Can you work these out from the drawing? Everything is in mm from the part's minimum corner. A direction names the side the tool comes from. Round coordinates to 2 decimals unless told otherwise and drop trailing zeros. Write each loop counter-clockwise with the first axis right and the second up, starting at its lowest first coordinate (ties: lowest second). Pieces come first, ordered by that corner, then holes. Notation, with made-up numbers: M -24.75,-5.75 L 26.25,-5.75 A20 ccw 26.25,7.25 Z; hole C 42.25,54 d11. An arc over 180 degrees is marked long. Use a Markdown table: item, result. Add a question column.
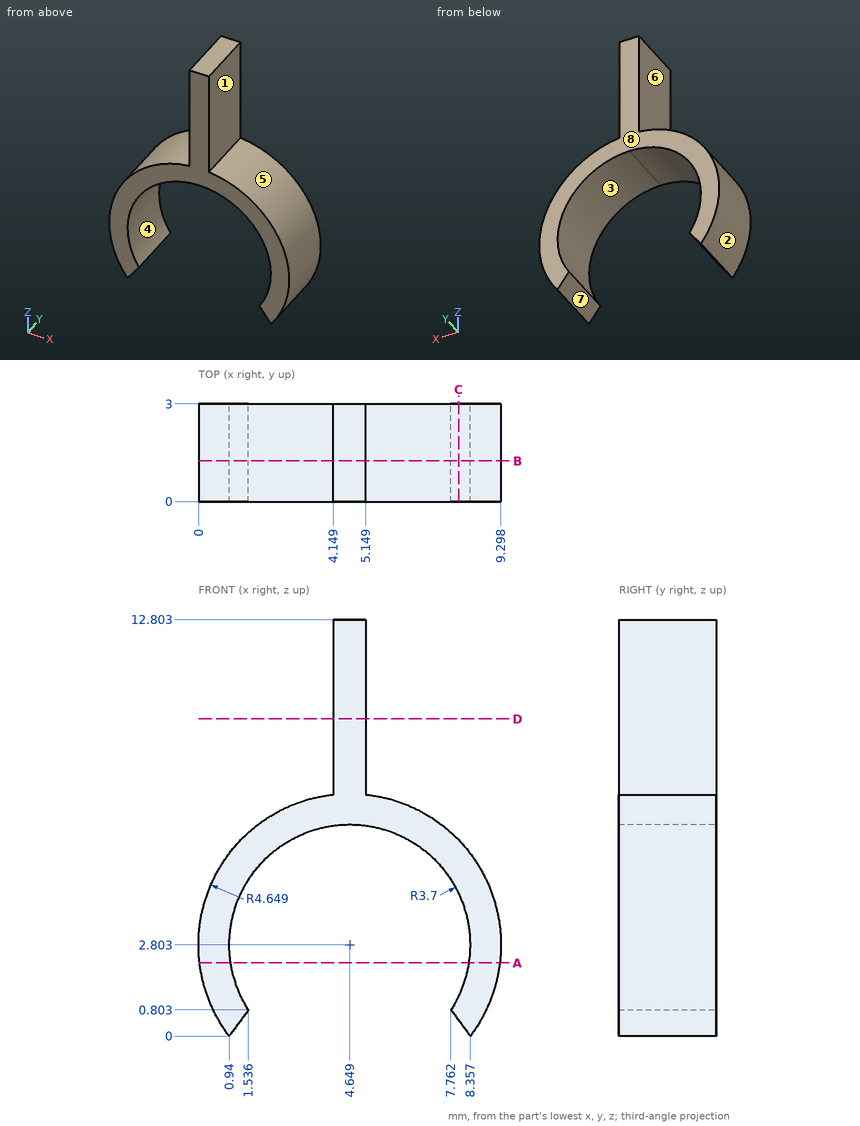
Item 1: Imagine slicing it at C-C on x = 8. List the corners of the cut face in (y, z) for me (1 decimal).
Item 2: I need wall thicknesses on probe 1 along X at (y, z) = (0.55, 8.5); probe 2 along X at (y, z) = (2.65, 4); probe 3 along X at (y, z) = (2.65, 4.75) (1 decimal). Which ranges of each line are inside material? Lowest first, please. Write a range as from..to.
Item 3: Imagine slicing it at D-D on z = 9.75. List the corners of the cut face in (x, y) for me.
Item 4: For pin 1 Ø2 at (x, z) = (7, 2.5) entering from -Y, with a flat end and sliding along its axis, tell me the tip position at first contact or that it passes through.
Item 5: Imagine slicing it at B-B on y = 1.25. List the corners of the cut face in (x, z) for me (1 decimal).
Item 6: Imagine slicing it at A-A on z = 2.25. List the corners of the cut face in (x, y) for me (1 decimal).
Item 7: On a 3-axis mill with a long thin cutter (end or side, diameter ignored), from which of +Z, -Z, +X, -X, +Y, -Y can I reach the whole of each face in a straight line? I mean the marked faces 4, 5, 6, 7 and 8. Say none if no direction works.
Item 8: If we mould it in two halves opening along X, with no side actions, what happens to the marked faces 1, 2 and 3? For each: +X half, -X half, draft (parallel to the pull), parting line (faces both ways), or undercut.
The answers:
| question | item | result |
|---|---|---|
| 1 | outline | M 0,0.5 L 3,0.5 L 3,1.2 L 0,1.2 Z; M 0,4.4 L 3,4.4 L 3,6 L 0,6 Z |
| 2 | probe 1 | 4.15..5.15 |
| 2 | probe 2 | 0.16..1.15, 8.15..9.14 |
| 2 | probe 3 | 0.4..1.5, 7.8..8.9 |
| 3 | outline | M 4.15,0 L 5.15,0 L 5.15,3 L 4.15,3 Z |
| 4 | pin 1 | through |
| 5 | outline | M 0.9,0 L 1.5,0.8 A3.7 cw 4.6,6.5 A3.7 cw 7.8,0.8 L 8.4,0 A4.6 ccw 5.1,7.4 L 5.1,12.8 L 4.1,12.8 L 4.1,7.4 A4.6 ccw Z |
| 6 | outline | M 0,0 L 1,0 L 1,3 L 0,3 Z; M 8.3,0 L 9.3,0 L 9.3,3 L 8.3,3 Z |
| 7 | face 4 | +Y, -Y |
| 7 | face 5 | +X, +Y, -Y |
| 7 | face 6 | +Z, -X, +Y, -Y |
| 7 | face 7 | -Z, +Y, -Y |
| 7 | face 8 | +Z, -Z, +X, -X, +Y |
| 8 | face 1 | +X half |
| 8 | face 2 | -X half |
| 8 | face 3 | undercut |
